Autodesk Inventor part; units mm, degrees
ref_plane "YZ Plane" through (0, 0, 0) normal (1, 0, 0) x (0, 1, 0)
ref_plane "XZ Plane" through (0, 0, 0) normal (0, 1, 0) x (-1, 0, 0)
ref_plane "XY Plane" through (0, 0, 0) normal (0, 0, 1) x (1, 0, 0)
sketch "Эскиз1" plane through (0, 0, 0) normal (0, 1, 0) x (-1, 0, 0)
  line L0 (0, 0) -> (77.5, 0)
  line L1 (77.5, 0) -> (77.5, -9)
  line L2 (77.5, -9) -> (55, -9)
  line L3 (55, -9) -> (55, -15)
  line L4 (0, -4) -> (0, 0)
  line L5 (55, -15) -> (45, -15)
  line L6 (45, -15) -> (45, -4)
  line L7 (45, -4) -> (0, -4)
  dimension "d0" = 155
  dimension "d1" = 110
  dimension "d3" = 9
  dimension "d5" = 15
  dimension "d6" = 90
  dimension "d7" = 4
revolve "Вращение1" add sketch "Эскиз1" angle 360 about axis through (0, 0, -4) along (0, 0, 1)
sketch "Эскиз3" plane through (0, 0, 0) normal (0, 0, 1) x (1, 0, 0)
  circle A0 centre (0, 0) radius 66.25 construction
  line L0 (0, 0) -> (-70.023, -70.023) construction
  line L1 (0, 0) -> (99.0274, 0) construction
  point P0 (0, 0)
  point P1 (-46.8458, -46.8458)
  point P2 (46.8458, -46.8458)
  point P3 (46.8458, 46.8458)
  point P4 (-46.8458, 46.8458)
  dimension "d15" = 132.5
  dimension "d16" = 135
  dimension "d19" = 360
hole "Отверстие1" at (-46.8458, -46.8458, 0) at (46.8458, -46.8458, 0) at (46.8458, 46.8458, 0) at (-46.8458, 46.8458, 0) direction (0, 0, -1) diameter 8.376 end through all
chamfer "Фаска1" distance 2 angle 45 2 edges at (55, 0, -15) (77.5, 0, 0)
properties part number "МПСТ Крышка подшипника глухая 110" material "Сталь, углеродистая"
CAD build for the part. Positions are in the model's coordinates, mm. A direction names the side the tool comes from. Coordinates: 2 decimals unless noted, no trailing zeros. Loops run counter-clockwise (first coordinate to the right, second up) from the corner with the lowest first, then second, coordinate; pieces in that order, holes last. Notation, with made-up numbers: (1.25, 33.5) - (26.25, 33.5) arc R27 cw to (26.25, 60.5) - close; hole circle Ø10 at (48, -4). An arc over 180 degrees is marked (long way). Return JSON: item names as keys, results as strings.
1. Band-saw the part on A-A (y = 0). Give the cut face in (x, z), and give its area (3 significant figures).
Result:
{"outline": "(-77.5, -9) - (-55, -9) - (-55, -13) - (-53, -15) - (-45, -15) - (-45, -4) - (45, -4) - (45, -15) - (53, -15) - (55, -13) - (55, -9) - (77.5, -9) - (77.5, -2) - (75.5, 0) - (-75.5, 0) - (-77.5, -2) - close", "area": "1,060 mm2"}
2. Mould opens along Y. For faces 1 (the conical face through (-72.133, 22.716, -0.125)), 2 (the flat face through (24, 39, -15)), 3 (the cylindrical face through (-20.765, 39.923, -9.423)), 4 (the cylindrical face through (43.314, 44.594, -4.563)) say: released by +Y, released by -Y, zero draft, split by the parting line, or undercut.
Result:
{"face 1": "split by the parting line", "face 2": "zero draft", "face 3": "undercut", "face 4": "undercut"}
3. Drop flat-ended pins along their axis: pin 1 (7.5 mm diameter, centred on x = 46.85, y = 46.85, fed in from +Z); pin 2 (1 mm diameter, centred on y = 21.5, z = -3.5, fed in from +X); pin 3 (2 mm diameter, centred on x = 46, y = 39, fed in from -Z); pin 4 (2 mm diameter, centred on x = -19, z = -8.5, fed in from +Y). Give the stop position or say it passes through.
Result:
{"pin 1": "passes through", "pin 2": "stops at x = 74.6", "pin 3": "stops at z = -9", "pin 4": "stops at y = 75.38"}
4. 3-axis set-ups, long thin cutter, end or side, ignore diameter. For faces 5 (the cylindrical face through (11.923, -53.692, -11.028)), 6 (the cylindrical face through (16.8, -75.657, -5.549)): which of +Z, -Z, +X, -X, +Y, -Y reach the whole face in a straight line?
Result:
{"face 5": "-Z", "face 6": "+Z, -Z"}
5. Probe L1, parallel to Y at x = 0, z = -7; L2, parallel to Z at x = 68, y = 24; L3, parallel to Z at x = 28.5, y = -13. List the from-to ranges inside material, lowest first. Write a range as from..to.
Result:
{"L1": "y = -77.5..-45, 45..77.5", "L2": "z = -9..0", "L3": "z = -4..0"}
